Could you check a few things on this model? Use its own coordinates, in mm. A direction names the side the tool comes from. Coordinates: 2 decimals unless noted, no trailing zeros. Write each loop counter-clockwise with the first axis right and the second up, starting at its lowest first coordinate (ties: lowest second). Pieces come first, ordered by that corner, then holes. Notation, with made-up numbers: (6, 82) - (20, 82) arc R20 cw to (20, 95) - close; hole circle Ø3 at (-10, 80.25). An arc over 180 degrees is marked (long way). Answer as a JSON object with one key per item and string values. Group by question number.
1) If we section it at B-B (x = 3.75): Write out the boundary of the cut face in (y, z).
2) If we section it at D-D (x = 5): Write out the boundary of the cut face in (y, z), plus the area to 3 significant figures.
3) If we section it at A-A (z = 2.25): Write out the boundary of the cut face in (x, y).
4) If we section it at C-C (y = 0.8): Write out the boundary of the cut face in (x, z), plus the area to 3 significant figures.
5) Please list where these lines run through material, in increasing order: line 1 along X through (y, z) = (1.45, 0); line 2 along X through (y, z) = (0.5, -3.5); line 3 along Z through (x, y) = (-3, 0.35).
6) On a 3-axis mill with a long thin cutter (end or side, diameter ignored), from which of +Z, -Z, +X, -X, +Y, -Y can I reach the whole of each face in a straight line? I mean faces 1 (the flat face through (-3, 1.6, 4)), 2 (the flat face through (-0.886, 0.811, -4.899)), 3 (the flat face through (1, 1, -5)). Say none if no direction works.
```python
from build123d import *

# Parameters (mm, degrees)
SKETCH_1_R          = 6.1
SKETCH_1_R_2        = 4.1
EXTRUDE_1_DEPTH     = 1.6
CUT_EXTRUDE_1_DEPTH = 9.773824708


with BuildPart() as part:
    # Эскиз1 → Бобышка-Вытянуть1 (new body)
    with BuildSketch(Plane(origin=(0, 0, 0), x_dir=(1, 0, 0), z_dir=(0, 1, 0))):
        with Locations(Location((0, 0, 0), (0, 0, 270))):
            Circle(SKETCH_1_R)
        with Locations(Location((0, 0, 0), (0, 0, 270))):
            Circle(SKETCH_1_R_2, mode=Mode.SUBTRACT)
    extrude(amount=EXTRUDE_1_DEPTH)

    # Эскиз2 → Вырез-Вытянуть1 (cut, through all)
    with BuildSketch(Plane.XY):
        Polygon((0, 0), (1.6, 1.6), (-0.097056275, 1.6), (-1.697056275, 0), align=None)
    extrude(amount=-CUT_EXTRUDE_1_DEPTH, mode=Mode.SUBTRACT)


solid = part.part
```
Here are the results:
{
 "1": {"outline": "(0, -4.81) - (1.6, -4.81) - (1.6, -1.66) - (0, -1.66) - close; (0, 1.66) - (1.6, 1.66) - (1.6, 4.81) - (0, 4.81) - close"},
 "2": {"outline": "(0, -3.49) - (1.6, -3.49) - (1.6, 3.49) - (0, 3.49) - close", "area": "11.2 mm²"},
 "3": {"outline": "(-5.67, 0) - (-3.43, 0) - (-3.43, 1.6) - (-5.67, 1.6) - close; (3.43, 0) - (5.67, 0) - (5.67, 1.6) - (3.43, 1.6) - close"},
 "4": {"outline": "(-0.9, -6.03) - (-0.9, -4) arc R4.1 cw (long way) to (0.8, -4.02) - (0.8, -6.05) arc R6.1 ccw (long way) to start", "area": "60.7 mm²"},
 "5": {"line 1": "x = -6.1 to -4.1, 4.1 to 6.1", "line 2": "x = -5 to -2.14, 2.14 to 5", "line 3": "z = -5.31 to -2.79, 2.79 to 5.31"},
 "6": {"face 1": "+Z, -Z, +X, -X, +Y", "face 2": "-Z, -Y", "face 3": "-Z, +Y"}
}
